Input: dimensioned drawing with shaded views. Units: mm. Origin: part minimum x, y, z. A direction names the side the tool comes from. Round coordinates to 2 decimals unless told otherwise and drop trailing zeros. Order: outer loops, then holes, each group sorted by start corner. A loop starts at its lowest first (then second) coordinate and runs counter-clockwise, first axis right, second up. Notation, with made-up numbers: (52.5, 61.5) - (84.5, 61.5) arc R25 cw to (84.5, 91.5) - close; hole circle Ø4 at (21.5, 36.5). An arc over 180 degrees is marked (long way). Return JSON: item names as keys, results as strings. Group by question number.
1) Ray query, line 1 (X direction, y = 2.6, z = 8); line 2 (X direction, y = 35, z = 6); line 3 (Z direction, x = 5, y = 2.2). Return the intervals inside material, ascending. Write a range as from..to.
2) Access query for the marked faces 1, 2 and 3. Directions: +Z, -Z, +X, -X, +Y, -Y. A direction counts if a zero-diameter tool reaches every point of the face in a straight line with its end or side. Return the directions, or none.
3) Section D-D, the plane z = 13. Return loops of the section in (x, y).
4) Contact query for flat-ended pins moving along their axis: P1, Ø5, axis at y = 33.21, z = 8, coming from the -X side; P2, Ø8, axis at x = 30.5, z = 12, coming from the -Y side; P3, Ø4, axis at y = 22, z = 13, coming from the +X side; P4, Ø3.5, axis at y = 33.21, z = 8, coming from the +X side. Output: stop coordinate, or through.
5) Section C-C, the plane x = 25. Return loops of the section in (y, z).
6) Section A-A, the plane x = 37. Return loops of the section in (y, z).
7) Mould query, pull axis X, two halves, no side actions, for the marked faces 4, 5 and 6. Classes: pulls with the +X half, pulls with the -X half, needs draft (parallel to the pull), parting line crosses it, or undercut.
8) Section B-B, the plane y = 23. Return loops of the section in (x, z).
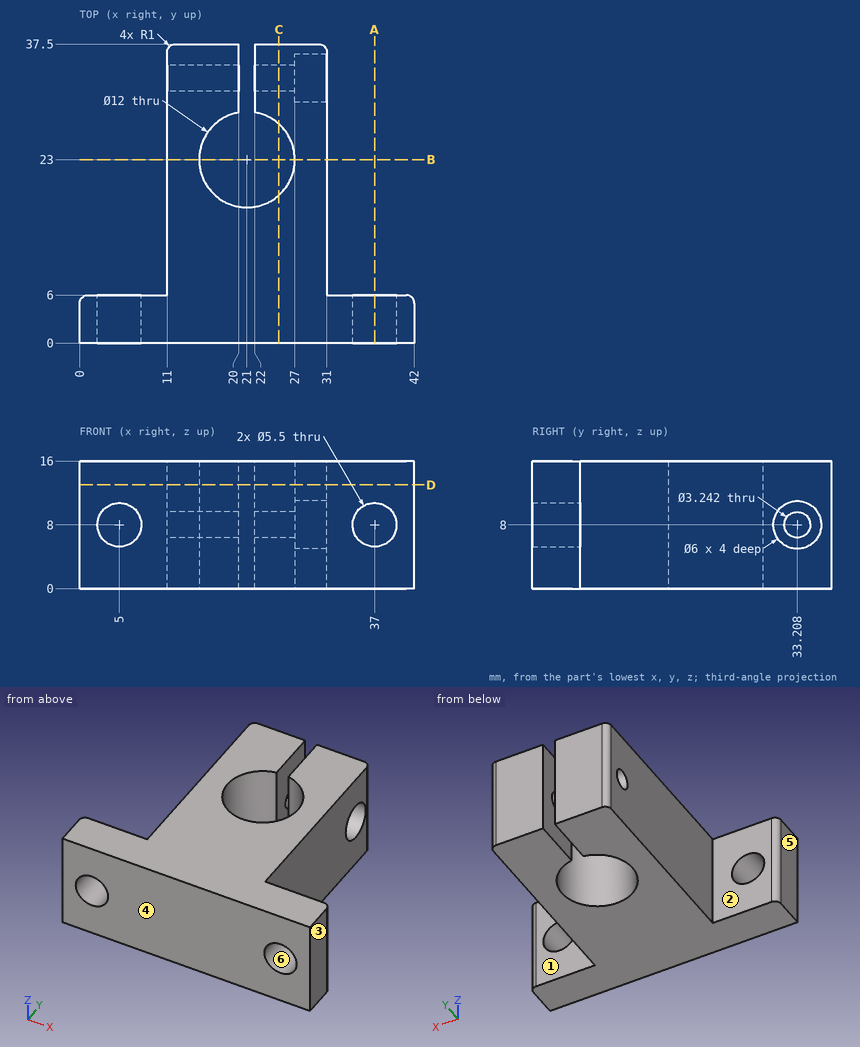
Geometry check:
{
 "1": {"line 1": "0..2.25, 7.75..34.25, 39.75..42", "line 2": "11..20, 22..27", "line 3": "0..5.25, 10.75..16"},
 "2": {"face 1": "+Z, -Z, +X, +Y", "face 2": "+Z, -Z, -X, +Y", "face 3": "+Z, -Z, +X, +Y, -Y"},
 "3": {"outline": "(0, 0) - (42, 0) - (42, 5) arc R1 ccw to (41, 6) - (31, 6) - (31, 36.5) arc R1 ccw to (30, 37.5) - (22, 37.5) - (22, 28.92) arc R6 cw (long way) to (20, 28.92) - (20, 37.5) - (12, 37.5) arc R1 ccw to (11, 36.5) - (11, 6) - (1, 6) arc R1 ccw to (0, 5) - close"},
 "4": {"P1": "x = 11", "P2": "y = 0", "P3": "x = 31", "P4": "x = 27"},
 "5": {"outline": "(0, 0) - (18.53, 0) - (18.53, 16) - (0, 16) - close; (27.47, 0) - (37.5, 0) - (37.5, 16) - (27.47, 16) - close; hole circle Ø3.24 at (33.21, 8)"},
 "6": {"outline": "(0, 0) - (6, 0) - (6, 5.25) - (0, 5.25) - close; (0, 10.75) - (6, 10.75) - (6, 16) - (0, 16) - close"},
 "7": {"face 4": "needs draft", "face 5": "pulls with the -X half", "face 6": "undercut"},
 "8": {"outline": "(11, 0) - (15, 0) - (15, 16) - (11, 16) - close; (27, 0) - (31, 0) - (31, 16) - (27, 16) - close"}
}
